Design review of the part built by this model. Coordinates are the model's own, in mm. A direction names the side the tool comes from. Give positions to 0.01 mm unless a question says otherwise; leave off trailing zeros. Loops run counter-clockwise (first coordinate to the right, second up) from the corner with the lowest first, then second, coordinate; pieces in that order, holes last. Notation, with made-up numbers: (56.25, 75.25) -> (108.25, 75.25) arc R19 cw to (108.25, 90.25) -> close; hole circle Ø3 at (38.5, -38.5). An arc over 180 degrees is marked (long way). Use CSV: the item, a comma, the result in double quotes. Start each with the question number.
Item 1: We need section D-D (x = 11). State the section outline as (y, z) points, plus the area to 3 significant figures.
Item 2: Clearance check with flat-ended pins moving along their axes: pin 1 (1.2 mm diameter, centred on x = -11.5, y = 2, fed in from +Z); pin 2 (1.2 mm diameter, centred on y = 3, z = -4.5, fed in from -X); pin 3 (1.9 mm diameter, centred on x = 0, z = -6, fed in from +Y). State where each tip first meets the part, or that it passes through.
Item 3: We need section B-B (y = 1.9). Count the separate pieces of the cut face and the enclosed holes in it, plus the area to 3 significant figures.
Item 4: We need section C-C (x = 6). State the section outline as (y, z) points (3 decimals).
Item 5: For faces 1 (the face through (15, 2, -47)), 2 (the face through (-13, 2, -10)), 3 (the face through (10, 2, -5)), list the 3-axis set-ups (+Z, -Z, +X, -X, +Y, -Y) from which the entire face can be reached by the end or side of a thin tool; tool diameter is ignored.
Item 6: Wall thickness on line 1 along Z through (x, y) = (1, 1.05); line 2 along X through (y, z) = (2.9, -84); line 3 along X through (y, z) = (2.05, -6) (3 decimals): over which ranges is each line inside the solid? List them lowest first. Write a range as from..to.
Item 7: The part is to be moulded in two halves that separate along Z. For faces 4 (the face through (-10, 2, -5)), 5 (the face through (1.55, 1.97, -79.09)), 6 (the face through (10.72, 2.03, -95.49)), say which applies: +Z half, -Z half, draft (parallel to the pull), parting line (faces both ways), or undercut.
Item 8: We need section A-A (z = -6). State the section outline as (x, y) points (3 decimals).
from build123d import *

# Parameters (mm, degrees)
SKETCH_1_R          = 1.625
SKETCH_1_R_2        = 5.15
EXTRUDE_1_DEPTH     = 4
FILLET_1_R          = 15
SKETCH_3_R          = 0.5
CUT_EXTRUDE_1_DEPTH = 102.197826064


with BuildPart() as part:
    # Эскиз1 → Бобышка-Вытянуть1 (new body)
    with BuildSketch(Plane(origin=(0, 0, 0), x_dir=(1, 0, 0), z_dir=(0, 1, 0))):
        Polygon((-10, 0), (10, 0), (10, 10), (15, 10), (15, 100), (-15, 100), (-15, 10), (-10, 10), align=None)
        with Locations(Location((-6, 15, 0), (0, 0, 270))):
            Circle(SKETCH_1_R, mode=Mode.SUBTRACT)
        with Locations(Location((0, 6, 0), (0, 0, 270))):
            Circle(SKETCH_1_R, mode=Mode.SUBTRACT)
        with Locations(Location((6, 15, 0), (0, 0, 90))):
            Circle(SKETCH_1_R, mode=Mode.SUBTRACT)
        with Locations(Location((0, 84, 0), (0, 0, 270))):
            Circle(SKETCH_1_R_2, mode=Mode.SUBTRACT)
    extrude(amount=EXTRUDE_1_DEPTH)

    # Скругление1
    fillet_1_edges = [part.edges().sort_by_distance(p)[0] for p in [
        (15, 2, -100),
        (-15, 2, -100),
    ]]
    fillet(fillet_1_edges, radius=FILLET_1_R - 0.0001)  # a hair under: the kernel refuses the full size

    # Эскиз3 → Вырез-Вытянуть1 (cut, through all)
    with BuildSketch(Plane(origin=(0, 4, 0), x_dir=(1, 0, 0), z_dir=(0, 1, 0))):
        with Locations(Location((0, 76.47, 0), (0, 0, 270))):
            Circle(SKETCH_3_R)
        with Locations(Location((0, 73.47, 0), (0, 0, 270))):
            Circle(SKETCH_3_R)
        with Locations(Location((0, 70.47, 0), (0, 0, 270))):
            Circle(SKETCH_3_R)
        with Locations(Location((0, 67.47, 0), (0, 0, 270))):
            Circle(SKETCH_3_R)
        with Locations(Location((0, 91.53, 0), (0, 0, 270))):
            Circle(SKETCH_3_R)
    extrude(amount=-CUT_EXTRUDE_1_DEPTH, mode=Mode.SUBTRACT)


solid = part.part
Results found:
1,outline,"(0, -95.2) -> (4, -95.2) -> (4, -10) -> (0, -10) -> close"
1,area,"341 mm²"
2,pin 1,"z = -10"
2,pin 2,"x = -10"
2,pin 3,"through"
3,separate pieces,"1"
3,enclosed holes,"9"
3,area,"2,690 mm²"
4,outline,"(0, -98.748) -> (4, -98.748) -> (4, -16.625) -> (0, -16.625) -> close; (0, -13.375) -> (4, -13.375) -> (4, 0) -> (0, 0) -> close"
5,face 1,"+Z, -Z, +X, +Y, -Y"
5,face 2,"+Z, -X, +Y, -Y"
5,face 3,"+Z, +X, +Y, -Y"
6,line 1,"-99.97..-89.05, -78.95..-7.28, -4.72..0"
6,line 2,"-15..-5.15, 5.15..15"
6,line 3,"-10..-1.625, 1.625..10"
7,face 4,"draft"
7,face 5,"undercut"
7,face 6,"-Z half"
8,outline,"(-10, 0) -> (-1.625, 0) -> (-1.625, 4) -> (-10, 4) -> close; (1.625, 0) -> (10, 0) -> (10, 4) -> (1.625, 4) -> close"
